from build123d import *

# Parameters (mm, degrees)
ESQUISSE1_R             = 2.046773471
BOSS_EXTRU_1_DEPTH      = 3.3
BOSS_EXTRU_2_DEPTH      = 1.3
BOSS_EXTRU_2_DEPTH_BACK = 4.6
ESQUISSE2_R             = 2.046773471
CHANFREIN1_SIZE         = 5
CHANFREIN1_SIZE_2       = 1.3
CHANFREIN3_SIZE         = 5
CHANFREIN3_SIZE_2       = 1.3
CHANFREIN2_SIZE         = 1
ESQUISSE3_R             = 5.5
ESQUISSE3_R_2           = 2.75
BOSS_EXTRU_3_DEPTH      = 1.8
CHANFREIN4_SIZE         = 1.5
ESQUISSE4_R             = 3.5
ENL_V_MAT_EXTRU_1_DEPTH = 3.5
CHANFREIN5_SIZE         = 1.3
ESQUISSE5_R             = 0.75
ENL_V_MAT_EXTRU_2_DEPTH = 3.5


with BuildPart() as part:
    # Esquisse1 → Boss.-Extru.1 (new body)
    with BuildSketch(Plane.XY):
        with BuildLine():
            Line((0.734265734, 6.96138304), (29.01958042, 3.977933166))
            ThreePointArc((29.01958042, 3.977933166), (32.6, 0), (29.01958042, -3.977933166))
            Line((29.01958042, -3.977933166), (0.734265734, -6.96138304))
            ThreePointArc((0.734265734, -6.96138304), (-7, 0), (0.734265734, 6.96138304))
        make_face()
        Circle(ESQUISSE1_R, mode=Mode.SUBTRACT)
    extrude(amount=BOSS_EXTRU_1_DEPTH)

    # Esquisse2 → Boss.-Extru.2 (add, two sides: drawn at the far end of the back side and taken through both)
    with BuildSketch(Plane.XY.offset(3.3).offset(-BOSS_EXTRU_2_DEPTH_BACK)):
        with BuildLine():
            Line((0.734265734, 6.96138304), (6.5, 6.353230741))
            Line((6.5, 6.353230741), (6.5, -6.353230741))
            Line((6.5, -6.353230741), (0.734265734, -6.96138304))
            ThreePointArc((0.734265734, -6.96138304), (-7, 0), (0.734265734, 6.96138304))
        make_face()
        Circle(ESQUISSE2_R, mode=Mode.SUBTRACT)
    extrude(amount=BOSS_EXTRU_2_DEPTH + BOSS_EXTRU_2_DEPTH_BACK)

    # Chanfrein1
    # the kernel refuses this chamfer: 5, 1.3 mm, written as the material it adds along each edge
    with BuildSketch(Plane(origin=(6.5, 19.337751576, 3.3), x_dir=(0.9999530531472482, 0, -0.009689762716214913), z_dir=(0, -1, 0))) as chanfrein1_piece_1_section:
        Polygon((CHANFREIN1_SIZE * 0.999953053147, CHANFREIN1_SIZE * 0.00968976271621), (-CHANFREIN1_SIZE_2 * 0.00968976271621, CHANFREIN1_SIZE_2 * 0.999953053147), (0, 0), align=None)
    chanfrein1_piece_1 = extrude(amount=38.675503153, mode=Mode.PRIVATE)
    chanfrein1_piece_1 = split(chanfrein1_piece_1, bisect_by=Plane(origin=(8.862365218, 6.104055566, 3.683257133), z_dir=(-0.10489510489510492, -0.994483291447898, 0)), keep=Keep.TOP, mode=Mode.PRIVATE)
    chanfrein1_piece_1 = split(chanfrein1_piece_1, bisect_by=Plane(origin=(8.862365218, -6.104055566, 3.683257133), z_dir=(-0.10489510489510483, 0.9944832914478982, 0)), keep=Keep.TOP, mode=Mode.PRIVATE)
    chanfrein1_piece_1 = split(chanfrein1_piece_1, bisect_by=Plane(origin=(8.218527805, 0, 4.6), z_dir=(0, 0, -1)), keep=Keep.TOP, mode=Mode.PRIVATE)
    add(chanfrein1_piece_1)

    # Chanfrein3
    # the kernel refuses this chamfer: 5, 1.3 mm, written as the material it adds along each edge
    with BuildSketch(Plane(origin=(6.5, 19.337751576, 0), x_dir=(0.9999530531472482, 0, 0.009689762716214958), z_dir=(0, -1, 0))) as chanfrein3_piece_1_section:
        Polygon((CHANFREIN3_SIZE * 0.999953053147, -CHANFREIN3_SIZE * 0.00968976271621), (-CHANFREIN3_SIZE_2 * 0.00968976271621, -CHANFREIN3_SIZE_2 * 0.999953053147), (0, 0), align=None)
    chanfrein3_piece_1 = extrude(amount=38.675503153, mode=Mode.PRIVATE)
    chanfrein3_piece_1 = split(chanfrein3_piece_1, bisect_by=Plane(origin=(8.862365218, 6.104055566, -0.383257133), z_dir=(-0.10489510489499053, -0.9944832914479101, 0)), keep=Keep.TOP, mode=Mode.PRIVATE)
    chanfrein3_piece_1 = split(chanfrein3_piece_1, bisect_by=Plane(origin=(8.862365218, -6.104055566, -0.383257133), z_dir=(-0.10489510489499053, 0.9944832914479101, 0)), keep=Keep.TOP, mode=Mode.PRIVATE)
    chanfrein3_piece_1 = split(chanfrein3_piece_1, bisect_by=Plane(origin=(8.218527805, 0, -1.3), z_dir=(0, 0, 1)), keep=Keep.TOP, mode=Mode.PRIVATE)
    add(chanfrein3_piece_1)

    # Chanfrein2
    chanfrein2_edges = [part.edges().sort_by_distance(p)[0] for p in [
        (-7, 0, -1.3),
        (3.617132867, 6.65730689, -1.3),
        (3.617132867, -6.65730689, -1.3),
        (-7, 0, 4.6),
        (3.617132867, -6.65730689, 4.6),
        (3.617132867, 6.65730689, 4.6),
    ]]
    chamfer(chanfrein2_edges, length=CHANFREIN2_SIZE)

    # Esquisse3 → Boss.-Extru.3 (add)
    with BuildSketch(Plane(origin=(0, 0, -1.3), x_dir=(-1, 0, 0), z_dir=(0, 0, -1))):
        with Locations(Location((0, 0, 0), (0, 0, 180))):
            Circle(ESQUISSE3_R)
        Circle(ESQUISSE3_R_2, mode=Mode.SUBTRACT)
    extrude(amount=BOSS_EXTRU_3_DEPTH)

    # Chanfrein4
    chanfrein4_edges = [part.edges().sort_by_distance(p)[0] for p in [
        (-5.5, 0, -3.1),
    ]]
    chamfer(chanfrein4_edges, length=CHANFREIN4_SIZE)

    # Esquisse4 → Enlèv. mat.-Extru.1 (cut)
    with BuildSketch(Plane.XY.offset(4.6)):
        Circle(ESQUISSE4_R)
    extrude(amount=-ENL_V_MAT_EXTRU_1_DEPTH, mode=Mode.SUBTRACT)

    # Chanfrein5
    chanfrein5_edges = [part.edges().sort_by_distance(p)[0] for p in [
        (-3.5, 0, 4.6),
    ]]
    chamfer(chanfrein5_edges, length=CHANFREIN5_SIZE)

    # Esquisse5 → Enlèv. mat.-Extru.2 (cut)
    with BuildSketch(Plane.XY.offset(3.3)):
        with Locations((29, 0)):
            Circle(ESQUISSE5_R)
        with Locations((25.8, 0)):
            Circle(ESQUISSE5_R)
        with Locations((22.6, 0)):
            Circle(ESQUISSE5_R)
        with Locations((19.4, 0)):
            Circle(ESQUISSE5_R)
    extrude(amount=-ENL_V_MAT_EXTRU_2_DEPTH, mode=Mode.SUBTRACT)


solid = part.part
The listing builds one solid part. Answer for the finished solid, in the listing's coordinates (mm). A direction names the side the tool comes from. Round coordinates to 2 decimals unless told otherwise and drop trailing zeros. Loops run counter-clockwise (first coordinate to the right, second up) from the corner with the lowest first, then second, coordinate; pieces in that order, holes last. Notation, with made-up numbers: M 73.25,27 L 81.25,27 A11 cw 81.25,37 Z; hole C -35.5,64.25 d4. An arc over 180 degrees is marked long. Return JSON: item names as keys, results as strings.
Q1. The mould has two halves that part along Y. Classify faces 5 (the face through (9.035, 0.083, -0.641)), 6 (the face through (3.604, -6.149, 4.107)), 7 (the face through (1.952, 0.615, -0.117)), 8 (the face through (-1.19, 5.37, -1.45)): released by +Y, released by -Y, zero draft, split by the parting line, or undercut.
Results list:
{"face 5": "zero draft", "face 6": "released by -Y", "face 7": "undercut", "face 8": "split by the parting line"}
Q2. Find section A-A, the plane x = 19.5. Determine the outline of the cut face in (y, z), plus the area to 3 significant figures.
Results list:
{"outline": "M -4.98,0 L -0.74,0 L -0.74,3.3 L -4.98,3.3 Z; M 0.74,0 L 4.98,0 L 4.98,3.3 L 0.74,3.3 Z", "area": "28.0 mm2"}
Q3. Each of these flat-tipped pins is pushed along its axis until it touches: pin 1 Ø5.5 at (x, y) = (-1, 1) entering from +Z; pin 2 Ø2 at (y, z) = (0, -1.5) entering from -X; pin 3 Ø2.5 at (x, y) = (25.8, 0) entering from -Z. Where does it stop, or does it pass through?
Results list:
{"pin 1": "stops at z = 3.96", "pin 2": "stops at x = -6.8", "pin 3": "stops at z = 0"}
Q4. Which of the six approach directions +Z, -Z, +X, -X, +Y, -Y give full straight-line access (tool end or side, diameter ignored) to faces 1 (the face through (5.4, -1.7, -1.3)), 2 (the face through (9.035, 0.083, 3.941)), 3 (the face through (22, -1, 0)), 4 (the face through (2, -2, 1.1))?
Results list:
{"face 1": "-Z", "face 2": "+Z, +X, +Y, -Y", "face 3": "-Z, +X, +Y, -Y", "face 4": "+Z"}
Q5. Find the intervals of material crossed by line 1 along Y through (x, z) = (0, 2); line 2 along Y through (x, z) = (0, 0); line 3 along X through (y, z) = (-2.5, 2), in increasing order. Write a range as from..to.
Results list:
{"line 1": "y = -7..-3.5, 3.5..7", "line 2": "y = -7..-2.05, 2.05..7", "line 3": "x = -6.54..-2.45, 2.45..31.72"}
Q6. Find section C-C, the plane x = 25.8. Determine the outline of the cut face in (y, z), plus the area to 3 significant figures.
Results list:
{"outline": "M -4.32,0 L -0.75,0 L -0.75,3.3 L -4.32,3.3 Z; M 0.75,0 L 4.32,0 L 4.32,3.3 L 0.75,3.3 Z", "area": "23.5 mm2"}
Q7. Find section B-B, the plane y = 0. State how many separate pieces and enclosed holes the cut face has, plus the area to 3 significant figures.
Results list:
{"separate pieces": "6", "enclosed holes": "0", "area": "123 mm2"}
